Input: part model. Units: mm. Frame: model coordinates. A direction names the side the tool comes from. Give positions to 0.01 mm unless a question says otherwise; leave off trailing zeros. Write each loop counter-clockwise with the first axis right and the second up, starting at its lowest first coordinate (ties: lowest second). Pieces come first, ordered by that corner, then holes. Notation, with made-up numbers: M -35.5,87 L -2.5,87 A20 ccw -2.5,92 Z; hole C 56,48.5 d2. An arc over 180 degrees is marked long. Use CSV: the item, a comma, the result in double quotes. Start each with the question number.
from build123d import *

# Parameters (mm, degrees)
SKETCH_1_R          = 1.625
EXTRUDE_1_DEPTH     = 3
FILLET_1_R          = 10
SKETCH_3_R          = 1.75
CUT_EXTRUDE_1_DEPTH = 10
SKETCH_4_R          = 1.75
CUT_EXTRUDE_2_DEPTH = 10
SKETCH_5_R          = 1.75
CUT_EXTRUDE_3_DEPTH = 10
CUT_EXTRUDE_4_DEPTH = 10


with BuildPart() as part:
    # Эскиз1 → Бобышка-Вытянуть1 (new body)
    with BuildSketch(Plane.XY):
        with BuildLine():
            ThreePointArc((-32.5, -28.5), (-35.328427125, -35.328427125), (-28.5, -32.5))
            Line((-28.5, -32.5), (28.5, -32.5))
            ThreePointArc((28.5, -32.5), (35.328427125, -35.328427125), (32.5, -28.5))
            Line((32.5, -28.5), (32.5, 28.5))
            ThreePointArc((32.5, 28.5), (35.328427125, 35.328427125), (28.5, 32.5))
            Line((28.5, 32.5), (-28.5, 32.5))
            ThreePointArc((-28.5, 32.5), (-35.328427125, 35.328427125), (-32.5, 28.5))
            Line((-32.5, 28.5), (-32.5, -28.5))
        make_face()
        with Locations((-32.5, -32.5)):
            Circle(SKETCH_1_R, mode=Mode.SUBTRACT)
        with Locations((32.5, 32.5)):
            Circle(SKETCH_1_R, mode=Mode.SUBTRACT)
        with Locations((-32.5, 32.5)):
            Circle(SKETCH_1_R, mode=Mode.SUBTRACT)
        with Locations((32.5, -32.5)):
            Circle(SKETCH_1_R, mode=Mode.SUBTRACT)
    extrude(amount=EXTRUDE_1_DEPTH)

    # Скругление1
    fillet_1_edges = [part.edges().sort_by_distance(p)[0] for p in [
        (-32.5, -28.5, 1.5),
        (-32.5, 28.5, 1.5),
        (-28.5, 32.5, 1.5),
        (28.5, 32.5, 1.5),
        (32.5, 28.5, 1.5),
        (32.5, -28.5, 1.5),
        (28.5, -32.5, 1.5),
        (-28.5, -32.5, 1.5),
    ]]
    fillet(fillet_1_edges, radius=FILLET_1_R)

    # Эскиз3 → Вырез-Вытянуть1 (cut)
    with BuildSketch(Plane(origin=(0, 0, 0), x_dir=(-1, 0, 0), z_dir=(0, 0, -1))):
        with Locations((-17.5, 27.5)):
            Circle(SKETCH_3_R)
        with Locations(Location((17.5, 27.5, 0), (0, 0, 180))):
            Circle(SKETCH_3_R)
    extrude(amount=-CUT_EXTRUDE_1_DEPTH, mode=Mode.SUBTRACT)

    # Эскиз4 → Вырез-Вытянуть2 (cut)
    with BuildSketch(Plane(origin=(0, 0, 0), x_dir=(-1, 0, 0), z_dir=(0, 0, -1))):
        with Locations((-17.5, -20)):
            Circle(SKETCH_4_R)
        with Locations(Location((17.5, -20, 0), (0, 0, 180))):
            Circle(SKETCH_4_R)
    extrude(amount=-CUT_EXTRUDE_2_DEPTH, mode=Mode.SUBTRACT)

    # Эскиз5 → Вырез-Вытянуть3 (cut)
    with BuildSketch(Plane(origin=(0, 0, 0), x_dir=(-1, 0, 0), z_dir=(0, 0, -1))):
        with Locations((-10.3, -7.5)):
            Circle(SKETCH_5_R)
        with Locations(Location((10.3, -7.5, 0), (0, 0, 180))):
            Circle(SKETCH_5_R)
    extrude(amount=-CUT_EXTRUDE_3_DEPTH, mode=Mode.SUBTRACT)

    # Эскиз7 → Вырез-Вытянуть4 (cut)
    # profile 1 of 2: a face of its own
    with BuildSketch(Plane(origin=(0, 0, 0), x_dir=(-1, 0, 0), z_dir=(0, 0, -1))):
        with BuildLine():
            Line((-7.65, -3.2), (4.85, -3.2))
            ThreePointArc((4.85, -3.2), (7.148097039, -4.151902961), (8.1, -6.45))
            Line((8.1, -6.45), (8.1, -8.55))
            ThreePointArc((8.1, -8.55), (7.148097039, -10.848097039), (4.85, -11.8))
            Line((4.85, -11.8), (-7.65, -11.8))
            ThreePointArc((-7.65, -11.8), (-7.968198052, -11.668198052), (-8.1, -11.35))
            Line((-8.1, -11.35), (-8.1, -3.65))
            ThreePointArc((-8.1, -3.65), (-7.968198052, -3.331801948), (-7.65, -3.2))
        make_face()
        with BuildLine():
            ThreePointArc((-7.85, -11.35), (-7.791421356, -11.491421356), (-7.65, -11.55))
            Line((-7.65, -11.55), (4.85, -11.55))
            ThreePointArc((4.85, -11.55), (6.971320344, -10.671320344), (7.85, -8.55))
            Line((7.85, -8.55), (7.85, -6.45))
            ThreePointArc((7.85, -6.45), (6.971320344, -4.328679656), (4.85, -3.45))
            Line((4.85, -3.45), (-7.65, -3.45))
            ThreePointArc((-7.65, -3.45), (-7.791421356, -3.508578644), (-7.85, -3.65))
            Line((-7.85, -3.65), (-7.85, -11.35))
        make_face(mode=Mode.SUBTRACT)
    # profile 2 of 2: a face of its own
    with BuildSketch(Plane(origin=(0, 0, 0), x_dir=(-1, 0, 0), z_dir=(0, 0, -1))):
        with BuildLine():
            Line((-7.85, -3.65), (-7.85, -11.35))
            ThreePointArc((-7.85, -11.35), (-7.791421356, -11.491421356), (-7.65, -11.55))
            Line((-7.65, -11.55), (4.85, -11.55))
            ThreePointArc((4.85, -11.55), (6.971320344, -10.671320344), (7.85, -8.55))
            Line((7.85, -8.55), (7.85, -6.45))
            ThreePointArc((7.85, -6.45), (6.971320344, -4.328679656), (4.85, -3.45))
            Line((4.85, -3.45), (-7.65, -3.45))
            ThreePointArc((-7.65, -3.45), (-7.791421356, -3.508578644), (-7.85, -3.65))
        make_face()
    extrude(amount=-CUT_EXTRUDE_4_DEPTH, mode=Mode.SUBTRACT)


solid = part.part
Q1. First-contact query: pin 1 Ø1.5 at (y, z) = (-11, 1.5) entering from +X; pin 2 Ø1.5 at (y, z) = (-7, 1.5) entering from -X; pin 3 Ø0.9 at (x, z) = (0, 2) entering from -Y. Flat tips, straight axial feed; report the tip coordinate or a pass-through.
Q2. Set-up query: faces 1 (the flat face through (-8.1, -7, 1)), 2 (the cylindrical face through (26.43, 33.22, 1.52)), 3 (the cylindrical face through (26.43, -33.22, 1.52)), 4 (the flat face through (-32.5, 0, 1)). Return all of +Z, -Z, +X, -X, +Y, -Y with unobstructed straight access to the full face (end or side cutting, diameter ignored); none if empty.
Q3. Pull-direction query (Y, two-part tool) for faces 5 (the cylindrical face through (-26.53, 33.26, 1.52)), 6 (the flat face through (-1, 1, 0)), 7 (the cylindrical face through (-34.123, 32.571, 1.479)); classes: released by +Y, released by -Y, zero draft, split by the parting line, or undercut.
Q4. Material intervals for L1, parallel to Y at x = -17.5, z = 2.3; L2, parallel to Y at x = 10.3, z = 1.25; L3, parallel to X at y = 27, z = 1.35, sorted ascending. Write a range as [from, to].
Q5. Section B-B, the plane y = -20. Return the cut outline in (x, z), and give its area (3 significant figures).
Q6. Section A-A, the plane x = -17.5. Return the cut outline in (y, z).
Q7. Section D-D, the plane x = -1. Return the cut outline in (y, z).
Q8. Section C-C, the plane y = -7.5. Return the cut outline in (x, z).
Check result:
1,pin 1,"stops at x = 32.5"
1,pin 2,"stops at x = -32.5"
1,pin 3,"stops at y = -32.5"
2,face 1,"+Z, -Z"
2,face 2,"+Z, -Z, +Y"
2,face 3,"+Z, -Z, -Y"
2,face 4,"+Z, -Z, -X"
3,face 5,"released by +Y"
3,face 6,"zero draft"
3,face 7,"undercut"
4,L1,"y = [-32.5, -21.75], [-18.25, 25.75], [29.25, 32.5]"
4,L2,"y = [-32.5, -9.25], [-5.75, 32.5]"
4,L3,"x = [-33.47, -19.18], [-15.82, 15.82], [19.18, 33.47]"
5,outline,"M -32.5,0 L -19.25,0 L -19.25,3 L -32.5,3 Z; M -15.75,0 L 15.75,0 L 15.75,3 L -15.75,3 Z; M 19.25,0 L 32.5,0 L 32.5,3 L 19.25,3 Z"
5,area,"174 mm²"
6,outline,"M -32.5,0 L -21.75,0 L -21.75,3 L -32.5,3 Z; M -18.25,0 L 25.75,0 L 25.75,3 L -18.25,3 Z; M 29.25,0 L 32.5,0 L 32.5,3 L 29.25,3 Z"
7,outline,"M -32.5,0 L -11.8,0 L -11.8,3 L -32.5,3 Z; M -3.2,0 L 32.5,0 L 32.5,3 L -3.2,3 Z"
8,outline,"M -32.5,0 L -12.05,0 L -12.05,3 L -32.5,3 Z; M -8.55,0 L -8.1,0 L -8.1,3 L -8.55,3 Z; M 8.1,0 L 8.55,0 L 8.55,3 L 8.1,3 Z; M 12.05,0 L 32.5,0 L 32.5,3 L 12.05,3 Z"
